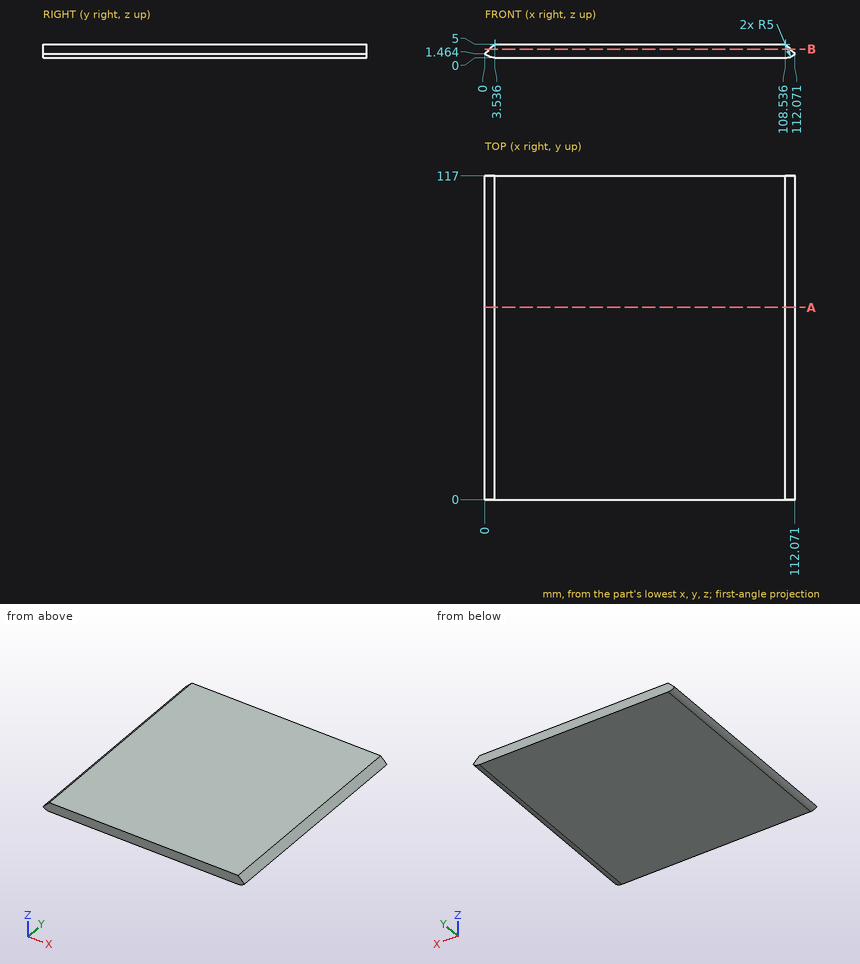
For this review, use the dimensioned drawing (mm, ordinates from the lowest corner) and the shaded views. Coordinates: 2 decimals unless noted, no trailing zeros. Order: outer loops, then holes, each group sorted by start corner. A loop starts at its lowest first (then second) coordinate and runs counter-clockwise, first axis right, second up. Notation, with made-up numbers: (17, 3) - (23, 3) arc R9 cw to (23, 11) - close; hole circle Ø6 at (79.5, 72). An arc over 180 degrees is marked (long way). Answer as a JSON object with one key per item and string values. Group by question number.
1. We need section B-B on z = 3.15. State the section outline as (x, y) points (1 decimal).
2. We need section A-A on y = 69.5. State the section outline as (x, z) points (1 decimal).
3. Clearance check with flat-ended pins moving along their axes: P1, Ø2, axis at y = 69.5, z = 0.5, coming from the -X side; P2, Ø1, axis at y = 101, z = 2, coming from the +X side (1 decimal). State where each tip first meets the part, or that it passes through.
4. For probe 1 along X at (y, z) = (24, 0.5) (1 decimal); probe 2 along X at (y, z) = (66.5, 0.4) (1 decimal), list the stretches that pass through material, from the lowest coordinate up.
Final values:
{
 "1": {"outline": "(1.7, 0) - (110.4, 0) - (110.4, 117) - (1.7, 117) - close"},
 "2": {"outline": "(0, 1.5) arc R5 ccw to (3.5, 0) - (108.5, 0) arc R5 ccw to (112.1, 1.5) - (108.5, 5) - (3.5, 5) - close"},
 "3": {"P1": "x = 0", "P2": "x = 112"},
 "4": {"probe 1": "1.4 to 110.7", "probe 2": "1.6 to 110.5"}
}
